from build123d import *

# Parameters (mm, degrees)
PD_R               = 19.098593171
HALF_WIDTH_DEPTH   = 10.67
TEETH_START        = -10.67
TEETH_DEPTH        = 10.67
CIRPATTERN1_COUNT  = 24
SKETCH4_R          = 20.022921169
SKETCH4_R_2        = 16.668593171
CUT_EXTRUDE1_DEPTH = 28.900037957
SKETCH5_R          = 13.880990835
CUT_EXTRUDE2_DEPTH = 26.875333749


with BuildPart() as part:
    # PD → half width (new body)
    with BuildSketch(Plane.XY):
        Circle(PD_R)
    extrude(amount=HALF_WIDTH_DEPTH)

    # Sketch3 → Teeth (cut)
    with BuildSketch(Plane.XY.offset(10.67).offset(TEETH_START)):
        with BuildLine():
            Line((0, 18.228593171), (0.407100386, 18.228593171))
            ThreePointArc((0.407100386, 18.228593171), (0.733390757, 18.078654939), (0.832130423, 17.733405235))
            ThreePointArc((0.832130423, 17.733405235), (2.1104249, 16.030268615), (3.785966743, 17.344525307))
            ThreePointArc((3.785966743, 17.344525307), (3.970699136, 17.652455205), (4.324678302, 17.712834254))
            Line((4.324678302, 17.712834254), (4.717907078, 17.607468921))
            Line((4.717907078, 17.607468921), (4.943079647, 18.44782439))
            ThreePointArc((4.943079647, 18.44782439), (2.492866643, 18.935202059), (0, 19.098593171))
            Line((0, 19.098593171), (0, 18.228593171))
        make_face()
    teeth = extrude(amount=TEETH_DEPTH, mode=Mode.SUBTRACT)

    # CirPattern1: Teeth ×24 about axis
    cirpattern1_axis = Axis((0, 0, 0), (0, 0, 1))
    for i in range(1, CIRPATTERN1_COUNT):
        add(teeth.rotate(cirpattern1_axis, i * 360 / CIRPATTERN1_COUNT), mode=Mode.SUBTRACT)

    # Sketch4 → Cut-Extrude1 (cut, through all)
    with BuildSketch(Plane(origin=(0, 0, 0), x_dir=(-1, 0, 0), z_dir=(0, 0, -1))):
        Circle(SKETCH4_R)
        Circle(SKETCH4_R_2, mode=Mode.SUBTRACT)
    extrude(amount=-CUT_EXTRUDE1_DEPTH, mode=Mode.SUBTRACT)

    # Sketch5 → Cut-Extrude2 (cut, through all)
    with BuildSketch(Plane(origin=(0, 0, 0), x_dir=(-1, 0, 0), z_dir=(0, 0, -1))):
        Circle(SKETCH5_R)
    extrude(amount=-CUT_EXTRUDE2_DEPTH, mode=Mode.SUBTRACT)


solid = part.part
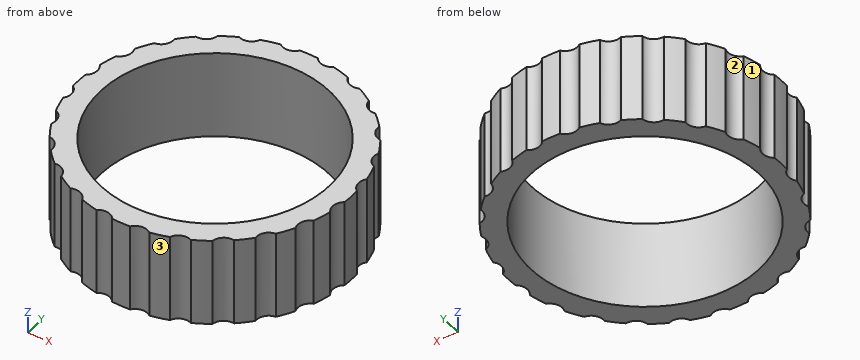
Read the model definition and answer for the solid it produces. Units are mm, in the model's axes. Face numbers are marked on the shaded views. Give positions to 0.01 mm unless a question says otherwise; leave off trailing zeros. Loops run counter-clockwise (first coordinate to the right, second up) from the corner with the lowest first, then second, coordinate; pieces in that order, holes last. Notation, with made-up numbers: M 78.5,71 L 99.5,71 A26 cw 99.5,109 Z; hole C -39,-14.5 d7. An arc over 180 degrees is marked long. Write each question's results on one line, items separated by ' | '.
1. Given pin 1 (3 mm diameter, centred on x = -0.5, z = 2.5, fed in from +Y); pin 2 (5 mm diameter, centred on x = -12, z = 4.5, fed in from +Y); pin 3 (3 mm diameter, centred on y = 2, z = 5.5, fed in from -X); pin 4 (3 mm diameter, centred on y = 9, z = 9, fed in from -X), each flat-ended and moving along its own axis, determine where each tip first touches the part or whether it passes through.
Values:
pin 1: stops at y = 16.67 | pin 2: stops at y = 13.2 | pin 3: stops at x = -16.66 | pin 4: stops at x = -14.89
2. Straight lines are drawn through the part: line 1 (Y direction, x = 0, z = 3); line 2 (Y direction, x = 1, z = 2); line 3 (X direction, y = -6.5, z = 4). For each, find the intervals that lie inside material, in ascending order. Write a range as [from, to].
Values:
line 1: y = [-16.67, -13.88], [13.88, 16.67] | line 2: y = [-16.64, -13.84], [13.84, 16.64] | line 3: x = [-14.85, -12.27], [12.27, 14.85]
3. Section A-A on x = 0 is taken. Give the vertices of the cut face in (y, z).
Values:
outline: M -16.67,0 L -13.88,0 L -13.88,10.67 L -16.67,10.67 Z; M 13.88,0 L 16.67,0 L 16.67,10.67 L 13.88,10.67 Z
4. The mould has two halves that part along Y. Classify the marked faces 1, 2 and 3: pulls with the +Y half, pulls with the -Y half, needs draft (parallel to the pull), parting line crosses it, or undercut.
Values:
face 1: pulls with the +Y half | face 2: undercut | face 3: pulls with the -Y half
